```python
from build123d import *

# Parameters (mm, degrees)
BOSS_EXTRUDE1_DEPTH = 2.54
CHAMFER1_SIZE       = 1.905


with BuildPart() as part:
    # Sketch1 → Boss-Extrude1 (new body)
    with BuildSketch(Plane(origin=(0, 0, 0), x_dir=(1, 0, 0), z_dir=(0, 1, 0))):
        with BuildLine():
            Line((0, -5.08), (83.82, -5.08))
            ThreePointArc((83.82, -5.08), (102.505005172, 2.659582555), (110.244587728, 21.344587728))
            Line((110.244587728, 21.344587728), (110.244587728, 38.108587728))
            ThreePointArc((110.244587728, 38.108587728), (102.505005172, 56.7935929), (83.82, 64.533175456))
            Line((83.82, 64.533175456), (0, 64.533175456))
            ThreePointArc((0, 64.533175456), (-18.685005172, 56.7935929), (-26.424587728, 38.108587728))
            Line((-26.424587728, 38.108587728), (-26.424587728, 21.344587728))
            ThreePointArc((-26.424587728, 21.344587728), (-18.685005172, 2.659582555), (0, -5.08))
        make_face()
        with BuildLine():
            Line((0, 0), (83.82, 0))
            ThreePointArc((83.82, 0), (98.912902724, 6.251685004), (105.164587728, 21.344587728))
            Line((105.164587728, 21.344587728), (105.164587728, 38.108587728))
            ThreePointArc((105.164587728, 38.108587728), (98.912902724, 53.201490452), (83.82, 59.453175456))
            Line((83.82, 59.453175456), (0, 59.453175456))
            ThreePointArc((0, 59.453175456), (-15.092902724, 53.201490452), (-21.344587728, 38.108587728))
            Line((-21.344587728, 38.108587728), (-21.344587728, 21.344587728))
            ThreePointArc((-21.344587728, 21.344587728), (-15.092902724, 6.251685004), (0, 0))
        make_face(mode=Mode.SUBTRACT)
    extrude(amount=BOSS_EXTRUDE1_DEPTH)

    # Chamfer1
    chamfer1_edges = [part.edges().sort_by_distance(p)[0] for p in [
        (-15.092902724, 2.54, -6.251685004),
        (41.91, 2.54, 0),
        (98.912902724, 2.54, -6.251685004),
        (105.164587728, 2.54, -29.726587728),
        (98.912902724, 2.54, -53.201490452),
        (41.91, 2.54, -59.453175456),
        (-15.092902724, 2.54, -53.201490452),
        (-21.344587728, 2.54, -29.726587728),
    ]]
    chamfer(chamfer1_edges, length=CHAMFER1_SIZE)


solid = part.part
```
Input: part model. Units: mm. Frame: model coordinates. A direction names the side the tool comes from. Give positions to 0.01 mm unless a question says otherwise; leave off trailing zeros. Loops run counter-clockwise (first coordinate to the right, second up) from the corner with the lowest first, then second, coordinate; pieces in that order, holes last.
1) Section query A-A on x = 18.5. Return the cut outline in (y, z) (3 decimals).
A:
outline: (0, -64.533) - (2.54, -64.533) - (2.54, -61.358) - (0.635, -59.453) - (0, -59.453) - close; (0, 0) - (0.635, 0) - (2.54, 1.905) - (2.54, 5.08) - (0, 5.08) - close
2) Section query C-C on y = 2. Return the cut outline in (x, z) (3 decimals).
A:
outline: (-26.425, -38.109) arc R26.425 ccw to (0, -64.533) - (83.82, -64.533) arc R26.425 ccw to (110.245, -38.109) - (110.245, -21.345) arc R26.425 ccw to (83.82, 5.08) - (0, 5.08) arc R26.425 ccw to (-26.425, -21.345) - close; hole (-22.71, -38.109) arc R22.71 ccw to (0, -60.818) - (83.82, -60.818) arc R22.71 ccw to (106.53, -38.109) - (106.53, -21.345) arc R22.71 ccw to (83.82, 1.365) - (0, 1.365) arc R22.71 ccw to (-22.71, -21.345) - close
3) Reachability of faces 1 (the flat face through (110.245, 1, -30)), 2 (the cylindrical face through (99.08, 0.31, -53.03)), 3 (the conical face through (98.829, 0.754, -6.001)) from +Z, -Z, +X, -X, +Y, -Y: full face, straight path, thin tool, end or side. Return the list, or none.
A:
face 1: +Z, -Z, +X, +Y, -Y
face 2: +Y, -Y
face 3: +Y
4) Mould query, pull axis X, two halves, no side actions, for faces 4 (the flat face through (42, 0, 1)), 5 (the conical face through (99.163, 0.754, -53.118)), 6 (the flat face through (-26.425, 1, -30)). Classes: released by +X, released by -X, zero draft, split by the parting line, or undercut.
A:
face 4: zero draft
face 5: undercut
face 6: released by -X
5) Line query: L1, parallel to Z at x = 58, y = 0.6; L2, parallel to X at y = 0.2, z = -57; L3, parallel to Z at x = 96, y = 1.45. Output: solid intervals per line, ascending.
A:
L1: z = -64.53 to -59.45, 0 to 5.08
L2: x = -18.48 to -9.94, 93.76 to 102.3
L3: z = -61.56 to -56.62, -2.83 to 2.11
6) Section query B-B on z = -26. Return the cut outline in (x, y) (3 decimals), and give its area (3 significant figures).
A:
outline: (-26.425, 0) - (-21.345, 0) - (-21.345, 0.635) - (-23.25, 2.54) - (-26.425, 2.54) - close; (105.165, 0) - (110.245, 0) - (110.245, 2.54) - (107.07, 2.54) - (105.165, 0.635) - close
area: 22.2 mm2
